```python
from build123d import *

# Parameters (mm, degrees)
IZIM1_W                      = 50.7
IZIM1_H                      = 48.2
Y_KSEKLIK_EKSTR_ZYON1_DEPTH  = 26.7
IZIM2_R                      = 8.7
Y_KSEKLIK_EKSTR_ZYON2_DEPTH  = 0.5
Y_KSEKLIK_EKSTR_ZYON3_DEPTH  = 11.9
IZIM4_R                      = 16.5
Y_KSEKLIK_EKSTR_ZYON4_DEPTH  = 0.9
IZIM5_R                      = 18
Y_KSEKLIK_EKSTR_ZYON5_DEPTH  = 0.9
Y_KSEKLIK_EKSTR_ZYON6_DEPTH  = 36
Y_KSEKLIK_EKSTR_ZYON7_DEPTH  = 17
Y_KSEKLIK_EKSTR_ZYON8_START  = 17
Y_KSEKLIK_EKSTR_ZYON8_DEPTH  = 17
IZIM9_W                      = 14.75
IZIM9_H                      = 70
KES_EKSTR_ZYON1_DEPTH        = 30.160746911
IZIM10_W                     = 14.75
IZIM10_H                     = 70
KES_EKSTR_ZYON2_DEPTH        = 30.160746911
IZIM11_W                     = 50.7
IZIM11_H                     = 48.2
Y_KSEKLIK_EKSTR_ZYON9_DEPTH  = 9.3
Y_KSEKLIK_EKSTR_ZYON10_START = 20
Y_KSEKLIK_EKSTR_ZYON10_DEPTH = 20
IZIM13_W                     = 9.75
IZIM13_H                     = 10.2
Y_KSEKLIK_EKSTR_ZYON11_DEPTH = 26.5
Y_KSEKLIK_EKSTR_ZYON12_DEPTH = 42.2
Y_KSEKLIK_EKSTR_ZYON13_START = -42.2
Y_KSEKLIK_EKSTR_ZYON13_DEPTH = 42.2
IZIM16_W                     = 29
IZIM16_H                     = 34.79
Y_KSEKLIK_EKSTR_ZYON14_DEPTH = 9.9
Y_KSEKLIK_EKSTR_ZYON15_DEPTH = 8.5
Y_KSEKLIK_EKSTR_ZYON16_DEPTH = 8.5
IZIM19_W                     = 6.3
IZIM19_H                     = 0.8
Y_KSEKLIK_EKSTR_ZYON17_DEPTH = 12
DRAFT1_ANGLE                 = 50
IZIM20_W                     = 5
IZIM20_H                     = 7.5
IZIM21_W                     = 5
IZIM21_H                     = 7.5
IZIM22_W                     = 5
IZIM22_H                     = 7.5
IZIM23_W                     = 5
IZIM23_H                     = 7.5
IZIM24_W                     = 5.2
IZIM24_H                     = 2.6
M27_BO_LUKLU_DELIK1_D        = 30.291
M27_BO_LUKLU_DELIK1_DEPTH    = 33.249
M27_BO_LUKLU_DELIK2_D        = 30.291
M27_BO_LUKLU_DELIK2_DEPTH    = 33.249
FEDER1_START                 = -30
FEDER1_DEPTH                 = 9.75
PAH1_SIZE                    = 1.479
RADYUS1_R                    = 0.8
RADYUS2_R                    = 2
RADYUS3_R                    = 5
RADYUS4_R                    = 5.1
RADYUS5_R                    = 7
RADYUS6_R                    = 8.16
L_EK1_SCALE                  = 0.192


# Read off the part's stored shape, not the designer's step: Feder1
with BuildPart() as part:
    # Çizim1 → Yükseklik-Ekstrüzyon1 (new body)
    with BuildSketch(Plane(origin=(18, 0, 0), x_dir=(0, 0, -1), z_dir=(1, 0, 0))):
        with Locations((-0.35, 68.8)):
            Rectangle(IZIM1_W, IZIM1_H)
    extrude(amount=-Y_KSEKLIK_EKSTR_ZYON1_DEPTH)

    # Çizim2 → Yükseklik-Ekstrüzyon2 (add)
    with BuildSketch(Plane.XZ.offset(-44.7)):
        with Locations(Location((0, 0, 0), (0, 0, 180))):
            Circle(IZIM2_R)
    extrude(amount=Y_KSEKLIK_EKSTR_ZYON2_DEPTH)

    # Çizim3 → Yükseklik-Ekstrüzyon3 (add)
    with BuildSketch(Plane(origin=(0, 44.2, 0), x_dir=(1, 0, 0), z_dir=(0, 1, 0))):
        Polygon((-18, 10.392304845), (-18, -10.392304845), (0, -20.784609691), (18, -10.392304845), (18, 10.392304845), (0, 20.784609691), align=None)
    extrude(amount=-Y_KSEKLIK_EKSTR_ZYON3_DEPTH)

    # Çizim4 → Yükseklik-Ekstrüzyon4 (add)
    with BuildSketch(Plane.XZ.offset(-32.3)):
        with Locations(Location((0, 0, 0), (0, 0, 270))):
            Circle(IZIM4_R)
    extrude(amount=Y_KSEKLIK_EKSTR_ZYON4_DEPTH)

    # Çizim5 → Yükseklik-Ekstrüzyon5 (add)
    with BuildSketch(Plane(origin=(0, 31.4, 0), x_dir=(1, 0, 0), z_dir=(0, 1, 0))):
        with Locations(Location((0, 0, 0), (0, 0, 90))):
            Circle(IZIM5_R)
    extrude(amount=-Y_KSEKLIK_EKSTR_ZYON5_DEPTH)

    # Çizim6 → Yükseklik-Ekstrüzyon6 (add)
    with BuildSketch(Plane.XY.offset(18)):
        with BuildLine():
            Line((-13.564659966, -21), (13.564659966, -21))
            ThreePointArc((13.564659966, -21), (17.201870235, -18.14099392), (20.25, -14.660746911))
            Line((20.25, -14.660746911), (35, -14.660746911))
            Line((35, -14.660746911), (35, 30.5))
            Line((35, 30.5), (0, 30.5))
            Line((0, 30.5), (-35, 30.5))
            Line((-35, 30.5), (-35, -14.660746911))
            Line((-35, -14.660746911), (-20.25, -14.660746911))
            ThreePointArc((-20.25, -14.660746911), (-17.201870235, -18.14099392), (-13.564659966, -21))
        make_face()
    extrude(amount=-Y_KSEKLIK_EKSTR_ZYON6_DEPTH)

    # Çizim7 → Yükseklik-Ekstrüzyon7 (add)
    with BuildSketch(Plane(origin=(0, 0, -18), x_dir=(-1, 0, 0), z_dir=(0, 0, -1))):
        with BuildLine():
            Line((13.564659966, -21), (-13.564659966, -21))
            ThreePointArc((-13.564659966, -21), (-17.201870235, -18.14099392), (-20.25, -14.660746911))
            Line((-20.25, -14.660746911), (-35, -14.660746911))
            Line((-35, -14.660746911), (-35, 30.5))
            Line((-35, 30.5), (35, 30.5))
            Line((35, 30.5), (35, -14.660746911))
            Line((35, -14.660746911), (20.25, -14.660746911))
            ThreePointArc((20.25, -14.660746911), (17.201870235, -18.14099392), (13.564659966, -21))
        make_face()
    extrude(amount=Y_KSEKLIK_EKSTR_ZYON7_DEPTH)

    # Çizim8 → Yükseklik-Ekstrüzyon8 (add)
    with BuildSketch(Plane.XY.offset(18).offset(Y_KSEKLIK_EKSTR_ZYON8_START)):
        with BuildLine():
            Line((13.564659966, -21), (-13.564659966, -21))
            ThreePointArc((-13.564659966, -21), (-17.201870235, -18.14099392), (-20.25, -14.660746911))
            Line((-20.25, -14.660746911), (-35, -14.660746911))
            Line((-35, -14.660746911), (-35, 30.5))
            Line((-35, 30.5), (35, 30.5))
            Line((35, 30.5), (35, -14.660746911))
            Line((35, -14.660746911), (20.25, -14.660746911))
            ThreePointArc((20.25, -14.660746911), (17.201870235, -18.14099392), (13.564659966, -21))
        make_face()
    extrude(amount=-Y_KSEKLIK_EKSTR_ZYON8_DEPTH)

    # Çizim9 → Kes-Ekstrüzyon1 (cut)
    with BuildSketch(Plane.XZ.offset(14.660746911)):
        with Locations((27.625, 0)):
            Rectangle(IZIM9_W, IZIM9_H)
    extrude(amount=-KES_EKSTR_ZYON1_DEPTH, mode=Mode.SUBTRACT)

    # Çizim10 → Kes-Ekstrüzyon2 (cut)
    with BuildSketch(Plane.XZ.offset(14.660746911)):
        with Locations((-27.625, 0)):
            Rectangle(IZIM10_W, IZIM10_H)
    extrude(amount=-KES_EKSTR_ZYON2_DEPTH, mode=Mode.SUBTRACT)

    # Çizim11 → Yükseklik-Ekstrüzyon9 (add)
    with BuildSketch(Plane.ZY.offset(8.7)):
        with Locations((0.35, 68.8)):
            Rectangle(IZIM11_W, IZIM11_H)
    extrude(amount=Y_KSEKLIK_EKSTR_ZYON9_DEPTH)

    # Çizim12 → Yükseklik-Ekstrüzyon10 (add)
    with BuildSketch(Plane.XY.offset(35).offset(Y_KSEKLIK_EKSTR_ZYON10_START)):
        with BuildLine():
            Line((-20.25, -14.660746911), (-20.25, 17.715834237))
            ThreePointArc((-20.25, 17.715834237), (0, 22), (20.25, 17.715834237))
            Line((20.25, 17.715834237), (20.25, -14.660746911))
            ThreePointArc((20.25, -14.660746911), (17.201870235, -18.14099392), (13.564659966, -21))
            Line((13.564659966, -21), (-13.564659966, -21))
            ThreePointArc((-13.564659966, -21), (-17.201870235, -18.14099392), (-20.25, -14.660746911))
        make_face()
    extrude(amount=-Y_KSEKLIK_EKSTR_ZYON10_DEPTH)

    # Çizim13 → Yükseklik-Ekstrüzyon11 (add)
    with BuildSketch(Plane.XZ.offset(-15.5)):
        with Locations((25.125, 15.1)):
            Rectangle(IZIM13_W, IZIM13_H)
    extrude(amount=Y_KSEKLIK_EKSTR_ZYON11_DEPTH)

    # Çizim14 → Yükseklik-Ekstrüzyon12 (add)
    with BuildSketch(Plane(origin=(0, 89.9, 0), x_dir=(1, 0, 0), z_dir=(0, 1, 0))):
        with BuildLine():
            Line((-18, -8.717797887), (-18, 8.717797887))
            ThreePointArc((-18, 8.717797887), (-20, 0), (-18, -8.717797887))
        make_face()
    extrude(amount=-Y_KSEKLIK_EKSTR_ZYON12_DEPTH)

    # Çizim15 → Yükseklik-Ekstrüzyon13 (add)
    with BuildSketch(Plane.XZ.offset(-47.7).offset(Y_KSEKLIK_EKSTR_ZYON13_START)):
        with BuildLine():
            Line((18, 8.717797887), (18, -8.717797887))
            ThreePointArc((18, -8.717797887), (20, 0), (18, 8.717797887))
        make_face()
    extrude(amount=Y_KSEKLIK_EKSTR_ZYON13_DEPTH)

    # Çizim16 → Yükseklik-Ekstrüzyon14 (add)
    with BuildSketch(Plane.XY.offset(25.7)):
        with Locations((0, 75.495)):
            Rectangle(IZIM16_W, IZIM16_H)
    extrude(amount=Y_KSEKLIK_EKSTR_ZYON14_DEPTH)

    # Çizim17 → Yükseklik-Ekstrüzyon15 (add)
    with BuildSketch(Plane.XY.offset(35.6)):
        Polygon((-9.4, 81.4), (-7.6, 81.4), (-7.6, 80.6), (-8.6, 80.6), (-8.6, 77.4), (-7.6, 77.4), (-7.6, 76.6), (-9.4, 76.6), align=None)
    extrude(amount=Y_KSEKLIK_EKSTR_ZYON15_DEPTH)

    # Çizim18 → Yükseklik-Ekstrüzyon16 (add)
    with BuildSketch(Plane.XY.offset(35.6)):
        Polygon((7.6, 77.4), (8.6, 77.4), (8.6, 80.6), (7.6, 80.6), (7.6, 81.4), (9.4, 81.4), (9.4, 76.6), (7.6, 76.6), align=None)
    extrude(amount=Y_KSEKLIK_EKSTR_ZYON16_DEPTH)

    # Çizim19 → Yükseklik-Ekstrüzyon17 (add)
    with BuildSketch(Plane.XY.offset(35.6)):
        with Locations((0, 70)):
            Rectangle(IZIM19_W, IZIM19_H)
    extrude(amount=Y_KSEKLIK_EKSTR_ZYON17_DEPTH)

    # Draft1
    draft1_faces = [part.faces().sort_by_distance(p)[0] for p in [
        (25.125, 2.25, 10),
    ]]
    draft(draft1_faces, Plane(origin=(0, -11, 0), x_dir=(0, 0, -1), z_dir=(0, -1, 0)), DRAFT1_ANGLE)

    # Çizim20 → Döndür1 (revolve)
    with BuildSketch(Plane.XY.offset(26.25), mode=Mode.PRIVATE) as d_nd_r1_sk:
        with Locations((-23.75, 34.25)):
            Rectangle(IZIM20_W, IZIM20_H)
    revolve(d_nd_r1_sk.sketch.rotate(Axis((-26.25, 38, 26.25), (0, -1, 0)), 270), axis=Axis((-26.25, 38, 26.25), (0, -1, 0)))

    # Çizim21 → Döndür2 (revolve)
    with BuildSketch(Plane.XY.offset(-26.25), mode=Mode.PRIVATE) as d_nd_r2_sk:
        with Locations((-23.75, 34.25)):
            Rectangle(IZIM21_W, IZIM21_H)
    revolve(d_nd_r2_sk.sketch.rotate(Axis((-26.25, 38, -26.25), (0, -1, 0)), 270), axis=Axis((-26.25, 38, -26.25), (0, -1, 0)))

    # Çizim22 → Döndür3 (revolve)
    with BuildSketch(Plane.XY.offset(-26.25), mode=Mode.PRIVATE) as d_nd_r3_sk:
        with Locations((28.75, 34.25)):
            Rectangle(IZIM22_W, IZIM22_H)
    revolve(d_nd_r3_sk.sketch.rotate(Axis((26.25, 38, -26.25), (0, -1, 0)), 270), axis=Axis((26.25, 38, -26.25), (0, -1, 0)))

    # Çizim23 → Döndür4 (revolve)
    with BuildSketch(Plane.XY.offset(26.25), mode=Mode.PRIVATE) as d_nd_r4_sk:
        with Locations((28.75, 34.25)):
            Rectangle(IZIM23_W, IZIM23_H)
    revolve(d_nd_r4_sk.sketch.rotate(Axis((26.25, 38, 26.25), (0, -1, 0)), 270), axis=Axis((26.25, 38, 26.25), (0, -1, 0)))

    # Çizim24 → Döndür5 (revolve)
    with BuildSketch(Plane(origin=(0, 0, 0), x_dir=(-1, 0, 0), z_dir=(0, 0, -1)), mode=Mode.PRIVATE) as d_nd_r5_sk:
        with Locations((-2.6, 94.2)):
            Rectangle(IZIM24_W, IZIM24_H)
    revolve(d_nd_r5_sk.sketch.rotate(Axis((0, 92.9, 0), (0, 1, 0)), 90), axis=Axis((0, 92.9, 0), (0, 1, 0)))

    # M27 Boşluklu Delik1
    with Locations(Plane.XY.offset(55)):
        with Locations((0, 0)):
            Hole(M27_BO_LUKLU_DELIK1_D / 2, depth=M27_BO_LUKLU_DELIK1_DEPTH)

    # M27 Boşluklu Delik2
    with Locations(Plane(origin=(0, 0, -35), x_dir=(-1, 0, 0), z_dir=(0, 0, -1))):
        with Locations((0, 0)):
            Hole(M27_BO_LUKLU_DELIK2_D / 2, depth=M27_BO_LUKLU_DELIK2_DEPTH)

    # Feder1 outline → Feder1 (add)
    with BuildSketch(Plane.YZ.offset(FEDER1_START)):
        Polygon((15.5, 19.826070485), (-9.313312955, 19.826070485), (-12.686687045, 12.591846402), (15.5, -20.999739147), align=None)
    extrude(amount=FEDER1_DEPTH)

    # Pah1
    pah1_edges = [part.edges().sort_by_distance(p)[0] for p in [
        (15.1455, 0, 55),
        (-15.1455, 0, -35),
    ]]
    chamfer(pah1_edges, length=PAH1_SIZE)

    # Radyus1
    radyus1_edges = [part.edges().sort_by_distance(p)[0] for p in [
        (-9.4, 81.4, 39.85),
        (-9.4, 76.6, 39.85),
        (9.4, 76.6, 39.85),
        (9.4, 81.4, 39.85),
    ]]
    fillet(radyus1_edges, radius=RADYUS1_R)

    # Radyus2
    radyus2_edges = [part.edges().sort_by_distance(p)[0] for p in [
        (-18, 68.8, -25),
        (-18, 68.8, 25.7),
        (-14.5, 92.89, 30.65),
        (-14.5, 58.1, 30.65),
        (14.5, 58.1, 30.65),
        (14.5, 92.89, 30.65),
        (18, 68.8, 25.7),
        (18, 68.8, -25),
    ]]
    fillet(radyus2_edges, radius=RADYUS2_R)

    # Radyus3
    radyus3_edges = [part.edges().sort_by_distance(p)[0] for p in [
        (-18, 38.25, -10.392304845),
        (0, 38.25, -20.784609691),
        (18, 38.25, -10.392304845),
        (18, 38.25, 10.392304845),
        (0, 38.25, 20.784609691),
        (-18, 38.25, 10.392304845),
    ]]
    fillet(radyus3_edges, radius=RADYUS3_R)

    # Radyus4
    radyus4_edges = [part.edges().sort_by_distance(p)[0] for p in [
        (25.125, -11, 20.2),
    ]]
    fillet(radyus4_edges, radius=RADYUS4_R)

    # Radyus5
    radyus5_edges = [part.edges().sort_by_distance(p)[0] for p in [
        (35, 23, 35),
        (-35, 23, -35),
        (35, 23, -35),
        (-35, 23, 35),
    ]]
    fillet(radyus5_edges, radius=RADYUS5_R)

    # Radyus6
    radyus6_edges = [part.edges().sort_by_distance(p)[0] for p in [
        (25.125, -11, 10),
    ]]
    fillet(radyus6_edges, radius=RADYUS6_R)


with BuildPart() as part_1:
    # Ölçek1: scaled about (0.014445195, 31.538640435, 4.897050437)
    add(part.part.scale(L_EK1_SCALE).moved(Location((0.011671718, 25.483221471, 3.956816753))))


solid = part_1.part
```
The model under review builds one solid part; all positions refer to its coordinate system, in mm. A direction names the side the tool comes from. Round coordinates to 2 decimals unless told otherwise and drop trailing zeros. Write each loop counter-clockwise with the first axis right and the second up, starting at its lowest first coordinate (ties: lowest second). Pieces come first, ordered by that corner, then holes.
(1) We need section B-B on y = 38.25. Give the boundary of the cut face in (x, z), and give its area (3 significant figures).
(2) Machinability: for faces 1 (the cylindrical face through (0, 32.8, 7.8)), 2 (the cylindrical face through (-0.367, 28.366, 0.613)), 3 (the flat face through (2.796, 40, 10)), 4 (the cylindrical face through (-3.32, 32.81, 2.04)), which of the approach directions +Z, -Z, +X, -X, +Y, -Y give a long, thin tool a straight path to every point of the face, cutting with its end or side? Answer none if there is none.
(3) Insertion check: pin 1 (1.5 mm diameter, centred on x = -5, z = -0.5, fed in from +Y); pin 2 (0.6 mm diameter, centred on x = -5, y = 26, fed in from +Z); pin 3 (5 mm diameter, centred on x = 4.5, y = 41.5, fed in from -Z). Each pin has a flat end and moves straight along its axis. Give the tip position at first contact, or say it passes through.
(4) Mouldability with a two-part tool opening along Y and no side actions: class faces 5 (the flat face through (0, 43.318, 10)), 6 (the flat face through (0, 38.846, 12)), 7 (the flat face through (6.732, 30, 4)), 8 (the cylindrical face through (3.323, 22.009, 5.998)) as +Y half, -Y half, draft (parallel to the pull), parting line (faces both ways), or undercut.
(5) We need section A-A on z = 12.75. Give the boundary of the cut face in (x, y), and give its area (3 significant figures).
(6) We need section D-D on y = 33.5. Give the boundary of the cut face in (x, z).
(7) Wall thickness on L1, parallel to Y at x = 2.5, z = -0.5; L2, parallel to X at y = 38.5, z = 10; L3, parallel to X at y = 35, z = 6: over which ranges is each line inside the solid? List them lowest first.
(8) We need section C-C on z = 10.25. Give the boundary of the cut face in (x, y).
Findings below:
1. outline: (-3.44, -0.46) arc R0.38 ccw to (-3.06, -0.84) - (3.08, -0.84) arc R0.38 ccw to (3.47, -0.46) - (3.47, 2.28) arc R3.84 ccw to (3.47, 5.63) - (3.47, 8.51) arc R0.38 ccw to (3.08, 8.89) - (2.8, 8.89) - (2.8, 10.79) - (-2.77, 10.79) - (-2.77, 8.89) - (-3.06, 8.89) arc R0.38 ccw to (-3.44, 8.51) - (-3.44, 5.63) arc R3.84 ccw to (-3.44, 2.28) - close
1. area: 79.5 mm2
2. face 1: +Z
2. face 2: -Z
2. face 3: +Z, +X, +Y
2. face 4: -Z, -X
3. pin 1: stops at y = 32.78
3. pin 2: stops at z = 7.76
3. pin 3: stops at z = -0.84
4. face 5: +Y half
4. face 6: undercut
4. face 7: draft
4. face 8: -Y half
5. outline: (-3.88, 22.67) arc R4.8 ccw to (-2.59, 21.45) - (2.62, 21.45) arc R4.8 ccw to (3.9, 22.67) - (3.9, 28.88) arc R9.6 ccw to (-3.88, 28.88) - close; (-0.59, 38.85) - (0.62, 38.85) - (0.62, 39) - (-0.59, 39) - close; hole circle Ø5.82 at (0.01, 25.48)
5. area: 34.4 mm2
6. outline: (-3.44, 2.52) arc R0.96 ccw to (-2.96, 1.68) - (-0.47, 0.24) arc R0.96 ccw to (0.49, 0.24) - (2.99, 1.68) arc R0.96 ccw to (3.47, 2.52) - (3.47, 5.4) arc R0.96 ccw to (2.99, 6.23) - (0.49, 7.67) arc R0.96 ccw to (-0.47, 7.67) - (-2.96, 6.23) arc R0.96 ccw to (-3.44, 5.4) - close
7. L1: y = 21.45 to 23.98, 26.99 to 31.34, 34.07 to 43.32
7. L2: x = -2.77 to 2.8
7. L3: x = -3.44 to 3.47
8. outline: (-6.35, 28.46) - (-3.88, 28.46) - (-3.88, 22.67) arc R4.8 ccw to (-2.59, 21.45) - (2.62, 21.45) arc R4.8 ccw to (3.9, 22.67) - (3.9, 28.46) - (6.37, 28.46) - (6.37, 31.34) - (-6.35, 31.34) - close; (-2.77, 37.02) arc R0.38 ccw to (-2.39, 36.64) - (2.41, 36.64) arc R0.38 ccw to (2.8, 37.02) - (2.8, 42.93) arc R0.38 ccw to (2.41, 43.32) - (-2.39, 43.32) arc R0.38 ccw to (-2.77, 42.93) - close; hole circle Ø5.82 at (0.01, 25.48)
